```python
from build123d import *

# Parameters (mm, degrees)
F1_DEPTH = 39


with BuildPart() as f1:
    # F0 (on Front) → F1 (new body)
    with BuildSketch(Plane.XZ):
        with BuildLine():
            ThreePointArc((65.9112834496, -35.7869070195), (0, 75), (-65.9112834496, -35.7869070195))
            Line((-65.9112834496, -35.7869070195), (-26.9968870374, -107.4583093791))
            ThreePointArc((-26.9968870374, -107.4583093791), (-23.2346773471, -132.5123240584), (-36.426916686, -154.1415333488))
            Line((-36.426916686, -154.1415333488), (-62.5, -175))
            ThreePointArc((-62.5, -175), (-65, -181.4384772072), (-62.5, -187.8769544143))
            ThreePointArc((-62.5, -187.8769544143), (0, -198), (62.5, -187.8769544143))
            ThreePointArc((62.5, -187.8769544143), (65, -181.4384772072), (62.5, -175))
            Line((62.5, -175), (36.426916686, -154.1415333488))
            ThreePointArc((36.426916686, -154.1415333488), (23.2346773471, -132.5123240584), (26.9968870374, -107.4583093791))
            Line((26.9968870374, -107.4583093791), (65.9112834496, -35.7869070195))
        make_face()
        with BuildLine():
            ThreePointArc((-34.7452932117, 38.6880420754), (-34.7452932117, 42.1772066019), (-32.6944137602, 45))
            ThreePointArc((-32.6944137602, 45), (-29.3760211009, 46.0782111348), (-26.0576284416, 45))
            ThreePointArc((-26.0576284416, 45), (0, 52), (26.0576284416, 45))
            ThreePointArc((26.0576284416, 45), (29.3760211009, 46.0782111348), (32.6944137602, 45))
            ThreePointArc((32.6944137602, 45), (34.7452932117, 42.1772066019), (34.7452932117, 38.6880420754))
            ThreePointArc((34.7452932117, 38.6880420754), (47.4908162017, 21.1807076486), (52, 0))
            ThreePointArc((52, 0), (51.7116488291, -5.4685807459), (50.8497932548, -10.8765125817))
            ThreePointArc((50.8497932548, -10.8765125817), (52.9006727063, -13.6993059798), (52.9006727063, -17.1884705063))
            ThreePointArc((52.9006727063, -17.1884705063), (50.8497932548, -20.0112639043), (47.5314005955, -21.0894750392))
            ThreePointArc((47.5314005955, -21.0894750392), (30.5648331192, -42.0688837075), (5.3692721108, -51.7220544546))
            ThreePointArc((5.3692721108, -51.7220544546), (3.3183926593, -54.5448478526), (0, -55.6230589875))
            ThreePointArc((0, -55.6230589875), (-3.3183926593, -54.5448478526), (-5.3692721108, -51.7220544546))
            ThreePointArc((-5.3692721108, -51.7220544546), (-30.5648331192, -42.0688837075), (-47.5314005955, -21.0894750392))
            ThreePointArc((-47.5314005955, -21.0894750392), (-50.8497932548, -20.0112639043), (-52.9006727063, -17.1884705063))
            ThreePointArc((-52.9006727063, -17.1884705063), (-52.9006727063, -13.6993059798), (-50.8497932548, -10.8765125817))
            ThreePointArc((-50.8497932548, -10.8765125817), (-49.4549388473, 16.0688837075), (-34.7452932117, 38.6880420754))
        make_face(mode=Mode.SUBTRACT)
        with BuildLine():
            ThreePointArc((26.0576284416, 45), (0, 52), (-26.0576284416, 45))
            Line((-26.0576284416, 45), (26.0576284416, 45))
        make_face()
        with BuildLine():
            Line((-50.8497932548, -10.8765125817), (-34.7452932117, 38.6880420754))
            ThreePointArc((-34.7452932117, 38.6880420754), (-49.4549388473, 16.0688837075), (-50.8497932548, -10.8765125817))
        make_face()
        with BuildLine():
            ThreePointArc((52, 0), (47.4908162017, 21.1807076486), (34.7452932117, 38.6880420754))
            Line((34.7452932117, 38.6880420754), (50.8497932548, -10.8765125817))
            ThreePointArc((50.8497932548, -10.8765125817), (51.7116488291, -5.4685807459), (52, 0))
        make_face()
        with BuildLine():
            Line((-5.3692721108, -51.7220544546), (-47.5314005955, -21.0894750392))
            ThreePointArc((-47.5314005955, -21.0894750392), (-30.5648331192, -42.0688837075), (-5.3692721108, -51.7220544546))
        make_face()
        with BuildLine():
            ThreePointArc((5.3692721108, -51.7220544546), (30.5648331192, -42.0688837075), (47.5314005955, -21.0894750392))
            Line((47.5314005955, -21.0894750392), (5.3692721108, -51.7220544546))
        make_face()
    extrude(amount=F1_DEPTH)


solid = f1.part
```
For this review, take the finished solid that the model builds, in its own axes (mm). A direction names the side the tool comes from. Coordinates: 2 decimals unless noted, no trailing zeros. Loops run counter-clockwise (first coordinate to the right, second up) from the corner with the lowest first, then second, coordinate; pieces in that order, holes last.
1. For line 1 (Z direction, x = 51.5, y = -12); line 2 (X direction, y = -6, z = 11); line 3 (X direction, y = -28, z = -49.5), list the stretches that pass through material, from the lowest coordinate up.
2. Insertion check: P1, Ø1.5, axis at y = -29.5, z = -113, coming from the -X side; P2, Ø12, axis at x = 2, y = -13, coming from the -Z side; P3, Ø1, axis at x = 47, y = -14.5, coming from the -Z side; P4, Ø2, axis at x = 4.5, y = -29.5, coming from the +Z side. Each pin has a flat end and moves straight along its axis. Give the tip position at first contact, or say it passes through.
3. Mouldability with a two-part tool opening along X and no side actions: class faces 6 (the cylindrical face through (2.17, -19.23, 74.97)), 7 (the flat face through (-46.726, -19.227, -71.121)), 8 (the flat face through (-42.91, -19.23, 13.56)), 9 (the flat face through (26.75, -19.23, -36.19)) as +X half, -X half, draft (parallel to the pull), parting line (faces both ways), or undercut.
4. Add section B-B, the plane x = -59. Give the boundary of the cut face in (y, z).
5. For faces 1 (the cylindrical face through (-0.89, -19.227, -197.998)), 2 (the flat face through (-1, 0, -60)), 3 (the flat face through (-49.281, -19.227, -164.425)), 4 (the flat face through (-26.155, -19.227, -36.62)), 5 (the flat face through (50, -19, -165)), list the 3-axis set-ups (+Z, -Z, +X, -X, +Y, -Y) from which the entire face can be reached by the end or side of a thin tool; tool diameter is ignored.
6. Add section C-C, the plane z = 0. Give the boundary of the cut face in (x, y).
7. Add section A-A, the plane y = -17.5. Give the boundary of the cut face in (x, z), then the cut area to 3 significant figures.
8. Add section D-D, the plane z = -158. Give the boundary of the cut face in (x, y), then the cut area to 3 significant figures.
Result:
1. line 1: z = -191.19 to -166.2, -62.33 to -19.46, -11.43 to 54.52
1. line 2: x = -74.19 to -43.74, 43.74 to 74.19
1. line 3: x = -58.47 to -8.43, 8.43 to 58.47
2. P1: stops at x = -24.82
2. P2: stops at z = -198
2. P3: stops at z = -192.46
2. P4: stops at z = 74.92
3. face 6: parting line
3. face 7: -X half
3. face 8: undercut
3. face 9: undercut
4. outline: (-39, -189.01) - (0, -189.01) - (0, -172.2) - (-39, -172.2) - close; (-39, -48.52) - (0, -48.52) - (0, 46.3) - (-39, 46.3) - close
5. face 1: -Z, +Y, -Y
5. face 2: +Z, -Z, +X, -X, +Y
5. face 3: -X, +Y, -Y
5. face 4: +Y, -Y
5. face 5: +X, +Y, -Y
6. outline: (-75, -39) - (-47.32, -39) - (-47.32, 0) - (-75, 0) - close; (47.32, -39) - (75, -39) - (75, 0) - (47.32, 0) - close
7. outline: (-65.91, -35.79) - (-27, -107.46) arc R37.11 cw to (-36.43, -154.14) - (-62.5, -175) arc R9.54 ccw to (-62.5, -187.88) arc R198 ccw to (62.5, -187.88) arc R9.54 ccw to (62.5, -175) - (36.43, -154.14) arc R37.11 cw to (27, -107.46) - (65.91, -35.79) arc R75 ccw (long way) to start; hole (-50.85, -10.88) arc R5.65 ccw to (-47.53, -21.09) - (-5.37, -51.72) arc R5.65 ccw to (5.37, -51.72) - (47.53, -21.09) arc R5.65 ccw to (50.85, -10.88) - (34.75, 38.69) arc R5.65 ccw to (26.06, 45) - (-26.06, 45) arc R5.65 ccw to (-34.75, 38.69) - close
7. area: 20,200 mm2
8. outline: (-41.25, -39) - (41.25, -39) - (41.25, 0) - (-41.25, 0) - close
8. area: 3,220 mm2
